Autodesk Inventor part; units mm, degrees
ref_plane "Work Plane1" through (0, 31.75, 0) normal (0, 1, 0) x (-1, 0, 0)
ref_plane "YZ Plane" through (0, 0, 0) normal (1, 0, 0) x (0, 1, 0)
ref_plane "XY Plane" through (0, 0, 0) normal (0, 0, 1) x (1, 0, 0)
sketch "Sketch2" plane through (0, 0, 0) normal (0, 1, 0) x (-1, 0, 0)
  circle A0 centre (0, 0) radius 3.175
  line L0 (0, 0) -> (35.56, 0)
  line L1 (0, 3.175) -> (12.2611, 3.175)
  line L2 (0, -3.175) -> (12.3047, -3.175)
  line L3 (13.1799, -3.1144) -> (35.56, 0)
  line L4 (35.56, 0) -> (13.1347, 3.1146)
  arc A1 (13.1347, 3.1146) -> (12.2611, 3.175) centre (12.2611, -3.175) ccw
  arc A2 (12.3047, -3.175) -> (13.1799, -3.1144) centre (12.3047, 3.175) ccw
  circle A3 centre (0, 0) radius 1.5875
  point P0 (12.7, 3.175)
  dimension "d5" = 6.35
  dimension "d6" = 35.56
  dimension "d7" = 12.7
  dimension "d8" = 6.35
  dimension "d9" = 6.35
  dimension "d12" = 3.175
ref_plane "Work Plane1" through (0, 31.75, 0) normal (0, 1, 0) x (-1, 0, 0)
sketch "Sketch3" plane through (0, 31.75, 0) normal (0, 1, 0) x (-1, 0, 0)
  circle A0 centre (0, 0) radius 1.5875
  line L0 (0, 1.5875) -> (12.4798, 1.5875)
  line L1 (0, -1.5875) -> (12.5018, -1.5875)
  line L2 (12.9421, -1.5722) -> (35.56, 0)
  line L3 (35.56, 0) -> (12.9197, 1.5722)
  arc A1 (12.9197, 1.5722) -> (12.4798, 1.5875) centre (12.4798, -4.7625) ccw
  arc A2 (12.5018, -1.5875) -> (12.9421, -1.5722) centre (12.5018, 4.7625) ccw
  point P0 (12.7, 1.5875)
  dimension "d14" = 3.175
  dimension "d15" = 12.7
  dimension "d16" = 6.35
  dimension "d17" = 6.35
loft "Loft1" add profiles "Sketch2", "Sketch3" contours A0 | L0 L3 A2 L2 A0 | A0 L1 A1 L4 L0 | A3 / all
sketch "Sketch4" plane through (0, 0, 0) normal (0, 0, 1) x (1, 0, 0)
  line L0 (-12.2611, 0) -> (0, 0)
  line L1 (0, 0) -> (0, 12.7)
  line L2 (0, 0) -> (0, 31.75)
  line L3 (0, 12.7) -> (-7.9375, 12.7)
  line L4 (-7.9375, 12.7) -> (-7.9375, 20.6375)
  arc A0 (0, 12.7) -> (-7.9375, 20.6375) centre (-7.9375, 12.7) ccw
  line L5 (-7.9375, 20.6375) -> (-14.2875, 20.6375)
  dimension "d22" = 12.7
  dimension "d23" = 7.9375
  dimension "d24" = 7.9375
  dimension "d25" = 6.35
sketch "Sketch5" plane through (-12.3047, 0, -3.175) normal (0, -1, 0) x (1, 0, 0)
  circle A0 centre (12.3047, 3.175) radius 1.7145
  dimension "d26" = 3.429
sweep "Sweep1" cut profiles "Sketch5" path "Sketch4" path curves L1 A0 L5
sketch "Sketch6" plane through (0, 0, 0) normal (0, 0, 1) x (1, 0, 0)
  line L0 (3.175, 0) -> (0, 0)
  line L1 (3.175, 0) -> (-3.175, 0)
  line L2 (0, 0) -> (-12.3047, 0)
  line L3 (-3.175, 0) -> (3.0911, 1.679)
  line L4 (3.175, 0) -> (1.5875, 31.75)
  dimension "d29" = 6.35
  dimension "d30" = 15
extrude "Extrusion3" cut sketch "Sketch6" along normal mid plane 25.4
properties part number "RudderLowerControlSurface"
Source: CAD feature listing. Evaluate the final solid. Frame: model axes, mm. A direction names the side the tool comes from. Round coordinates to 2 decimals unless told otherwise and drop trailing zeros. Use a Markdown table: item, result. Add a question column.
1. Mould query, pull axis Z, two halves, no side actions, for faces 1 (the conical face through (2.37, 16.08, -0.05)), 2 (the flat face through (-1.478, 0.455, 1.367)), 3 (the cylindrical face through (-11.157, 19.374, -1.159)). Classes: +Z half, -Z half, draft (parallel to the pull), parting line (faces both ways), or undercut.
2. Line query: probe 1 along Y at (x, z) = (-12, 0); probe 2 along Z at (x, y) = (0, 13) (1 decimal); probe 3 along Z at (x, y) = (-32.5, 13.5). Output: solid intervals per line, ascending.
3. First-contact query: pin 1 (4 mm diameter, centred on x = -14, y = 23, fed in from -Z); pin 2 (4 mm diameter, centred on x = -26, y = 15, fed in from -Z); pin 3 (10 mm diameter, centred on x = -27, y = 9, fed in from +Z). Flat tips, straight axial feed; report the tip coordinate or a pass-through.
4. Set-up query: faces 4 (the flat face through (-16, 0, 0)), 5 (the flat face through (-14.288, 21, 0)), 6 (the cylindrical face through (-1.713, 6.629, -0.075)). Return all of +Z, -Z, +X, -X, +Y, -Y with unobstructed straight access to the full face (end or side cutting, diameter ignored); none if empty.
Derived:
| question | item | result |
|---|---|---|
| 1 | face 1 | parting line |
| 1 | face 2 | draft |
| 1 | face 3 | undercut |
| 2 | probe 1 | 0 to 18.92, 22.35 to 31.75 |
| 2 | probe 2 | -2.5 to -1.7, 1.7 to 2.5 |
| 2 | probe 3 | -0.33 to 0.33 |
| 3 | pin 1 | z = -2.09 |
| 3 | pin 2 | z = -1.23 |
| 3 | pin 3 | z = 1.63 |
| 4 | face 4 | +Z, -Z, +X, -X, -Y |
| 4 | face 5 | none |
| 4 | face 6 | -Y |
